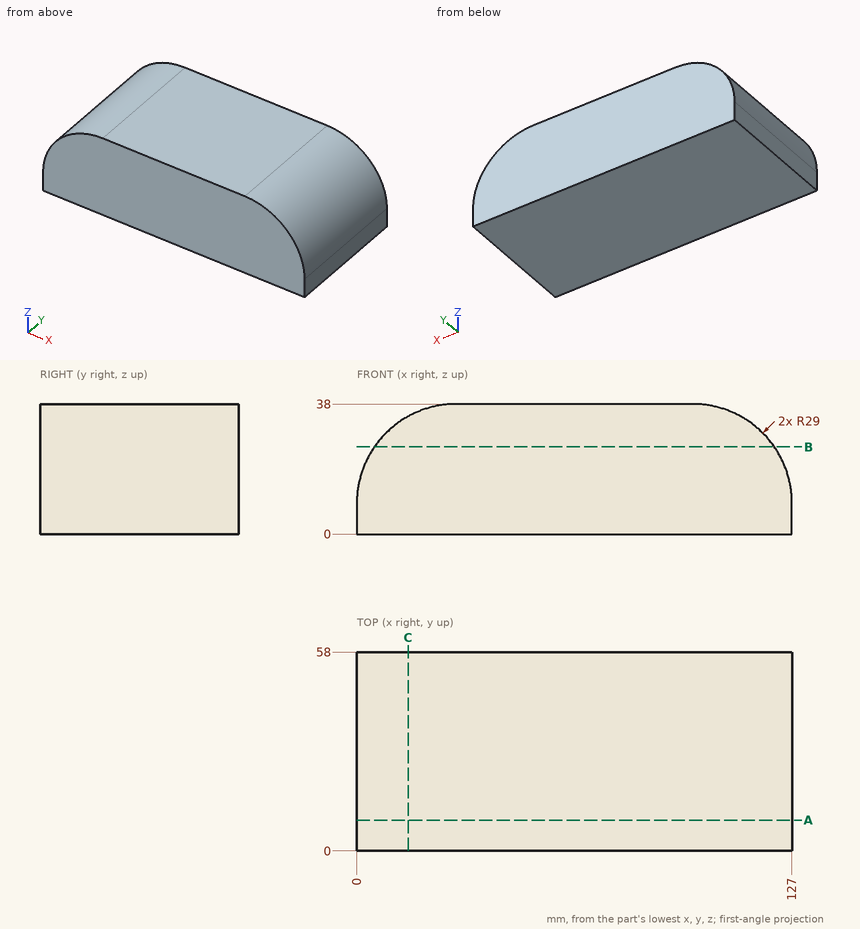
Check sheet for the drawn part. Datum: minimum x, y, z corner. Units: mm. Coordinates: 2 decimals unless noted, no trailing zeros. Write each loop counter-clockwise with the first axis right and the second up, starting at its lowest first coordinate (ties: lowest second). Pieces come first, ordered by that corner, then holes. Notation, with made-up numbers: (42, 16) - (93, 16) arc R18 ccw to (93, 38) - close; hole circle Ø9 at (19, -23). An arc over 180 degrees is marked (long way). Answer as a JSON object with one key per item and string values.
(1) Gauge pin test, flat end, axial feed: pin 1 Ø12 at (y, z) = (39.5, 18) entering from -X. Record the tip position at first contact, or that the pin passes through.
Report:
{"pin 1": "x = 0.16"}
(2) Cross-section at A-A on y = 9. Record the cut outline in (x, z), plus the area to 3 significant figures.
Report:
{"outline": "(0, 0) - (127, 0) - (127, 9) arc R29 ccw to (98, 38) - (29, 38) arc R29 ccw to (0, 9) - close", "area": "4,470 mm^2"}
(3) Cross-section at C-C on x = 15. Record the cut outline in (y, z).
Report:
{"outline": "(0, 0) - (58, 0) - (58, 34.4) - (0, 34.4) - close"}
(4) Cross-section at B-B on z = 25.5. Record the cut outline in (x, y), plus the area to 3 significant figures.
Report:
{"outline": "(5.15, 0) - (121.85, 0) - (121.85, 58) - (5.15, 58) - close", "area": "6,770 mm^2"}
(5) Thickness scan on line 1 along X through (y, z) = (12, 27.5); line 2 along X through (y, z) = (51.5, 20); line 3 along Z through (x, y) = (103, 38.5). Record the ranges inside material, lowest first.
Report:
{"line 1": "6.67 to 120.33", "line 2": "2.17 to 124.83", "line 3": "0 to 37.57"}
